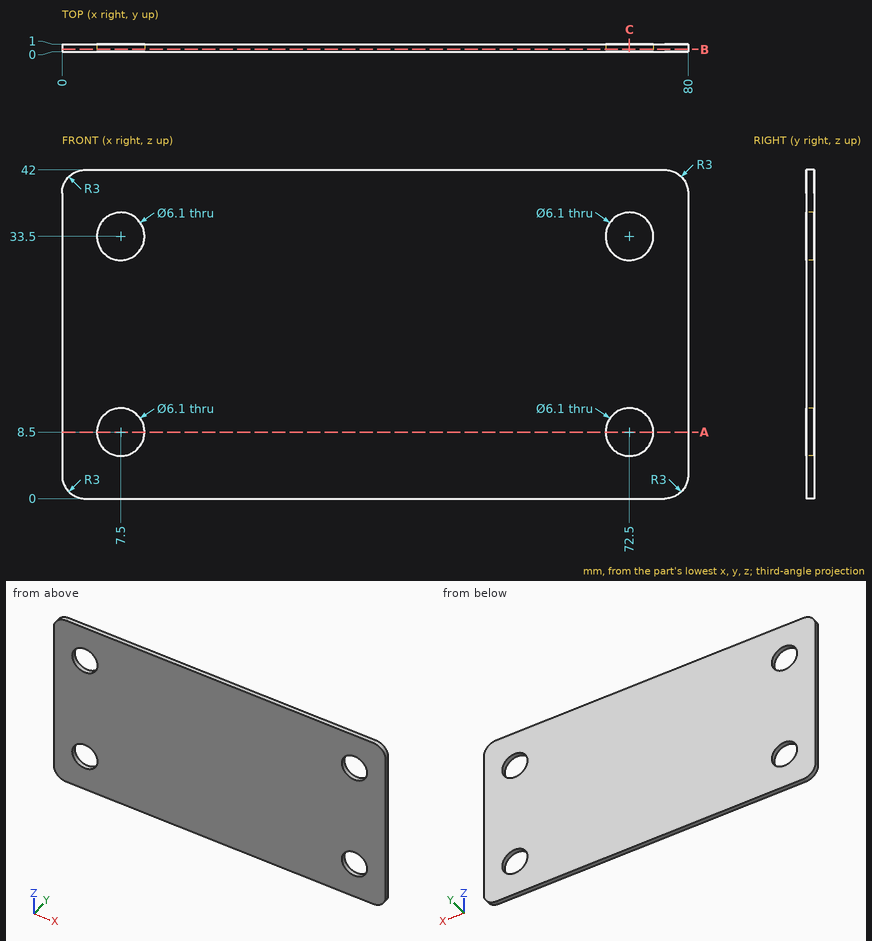
Geometry: see drawing. Coordinates: mm, zero at the bounding-box minimum. Give positions to 0.01 mm unless a question says otherwise; leave off trailing zeros. Order: outer loops, then holes, each group sorted by start corner. A loop starts at its lowest first (then second) coordinate and runs counter-clockwise, first axis right, second up. Notation, with made-up numbers: M 60,-38.75 L 116,-38.75 A27 cw 116,-7.75 Z; hole C 55,24 d3. An arc over 180 degrees is marked long. Answer as CSV lines item,"result". Start each with the question number.
1) Cut plane A-A (z = 8.5). Output: boundary loops of the cut face in (x, y).
2) Line query: line 1 (Z direction, x = 72.5, y = 0.7); line 2 (X direction, y = 0.3, z = 33.5); line 3 (Z direction, x = 9, y = 0.7). Output: solid intervals per line, ascending. Write a range as from..to.
3) Cut plane C-C (x = 72.5). Output: boundary loops of the cut face in (y, z).
4) Cut plane B-B (y = 0.3). Output: boundary loops of the cut face in (x, z), then the cut area to 3 significant figures.
Findings below:
1,outline,"M 0,0 L 4.45,0 L 4.45,1 L 0,1 Z; M 10.55,0 L 69.45,0 L 69.45,1 L 10.55,1 Z; M 75.55,0 L 80,0 L 80,1 L 75.55,1 Z"
2,line 1,"z = 0..5.45, 11.55..30.45, 36.55..42"
2,line 2,"x = 0..4.45, 10.55..69.45, 75.55..80"
2,line 3,"z = 0..5.84, 11.16..30.84, 36.16..42"
3,outline,"M 0,0 L 1,0 L 1,5.45 L 0,5.45 Z; M 0,11.55 L 1,11.55 L 1,30.45 L 0,30.45 Z; M 0,36.55 L 1,36.55 L 1,42 L 0,42 Z"
4,outline,"M 0,3 A3 ccw 3,0 L 77,0 A3 ccw 80,3 L 80,39 A3 ccw 77,42 L 3,42 A3 ccw 0,39 Z; hole C 7.5,8.5 d6.1; hole C 7.5,33.5 d6.1; hole C 72.5,8.5 d6.1; hole C 72.5,33.5 d6.1"
4,area,"3,240 mm²"
